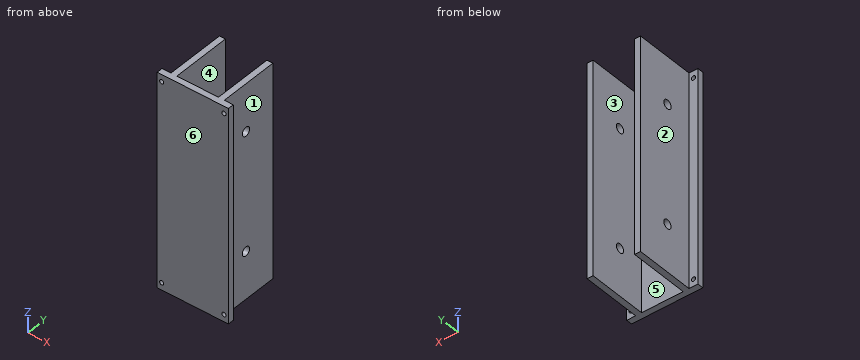
```python
from build123d import *

# Parameters (mm, degrees)
BOSS_EXTRUDE1_DEPTH = 228.6
SKETCH4_R           = 2.2479
CUT_EXTRUDE1_DEPTH  = 250.191994253
SKETCH5_R           = 4.7625
CUT_EXTRUDE2_DEPTH  = 249.158292477


with BuildPart() as part:
    # Sketch1 → Boss-Extrude1 (new body)
    with BuildSketch(Plane.XY):
        Polygon((0, 0), (76.2, 0), (76.2, 6.35), (66.675, 6.35), (66.675, 69.85), (60.325, 69.85), (60.325, 6.35), (15.875, 6.35), (15.875, 69.85), (9.525, 69.85), (9.525, 6.35), (0, 6.35), align=None)
    extrude(amount=BOSS_EXTRUDE1_DEPTH)

    # Sketch4 → Cut-Extrude1 (cut, through all)
    with BuildSketch(Plane(origin=(0, 6.35, 0), x_dir=(1, 0, 0), z_dir=(0, 1, 0))):
        with Locations(Location((4.7625, -7.62, 0), (0, 0, 180))):
            Circle(SKETCH4_R)
        with Locations(Location((4.7625, -220.98, 0), (0, 0, 180))):
            Circle(SKETCH4_R)
        with Locations((71.4375, -220.98)):
            Circle(SKETCH4_R)
        with Locations((71.4375, -7.62)):
            Circle(SKETCH4_R)
    extrude(amount=-CUT_EXTRUDE1_DEPTH, mode=Mode.SUBTRACT)

    # Sketch5 → Cut-Extrude2 (cut, through all)
    with BuildSketch(Plane(origin=(66.675, 0, 0), x_dir=(0, 0, -1), z_dir=(1, 0, 0))):
        with Locations(Location((-177.8, 34.676908919, 0), (0, 0, 90))):
            Circle(SKETCH5_R)
        with Locations(Location((-50.8, 34.676908919, 0), (0, 0, 90))):
            Circle(SKETCH5_R)
    extrude(amount=-CUT_EXTRUDE2_DEPTH, mode=Mode.SUBTRACT)


solid = part.part
```
Geometry: final body of the model. Coordinates: model frame, mm. Face numbers are marked on the shaded views. A direction names the side the tool comes from. Coordinates: 2 decimals unless noted, no trailing zeros. Order: outer loops, then holes, each group sorted by start corner. A loop starts at its lowest first (then second) coordinate and runs counter-clockwise, first axis right, second up. Notation, with made-up numbers: (37.5, -3.5) -> (52.5, -3.5) arc R12 cw to (52.5, 8.5) -> close; hole circle Ø5 at (16.25, -34). An arc over 180 degrees is marked (long way). Write each question's results on one line, items separated by ' | '. Start each with the question number.
1) Cut plane B-B, the plane y = 60. Output: boundary loops of the cut face in (x, z) (3 decimals), and give its area (3 significant figures).
2) First-contact query: pin 1 (5 mm diameter, centred on y = 53, z = 101.5, fed in from -X) (3 decimals); pin 2 (3 mm diameter, centred on x = 20.5, z = 74.5, fed in from +Y); pin 3 (12.5 mm diameter, centred on y = 34.68, z = 50.8, fed in from +X) (3 decimals). Flat tips, straight axial feed; report the tip coordinate or a pass-through.
3) Material intervals for line 1 along X through (y, z) = (3.25, 220.98); line 2 along X through (y, z) = (20, 94.5) (3 decimals); line 3 along Y through (x, z) = (6, 111), sorted ascending.
4) Cut plane D-D, the plane z = 7.62. Output: boundary loops of the cut face in (x, y) (3 decimals), and give its area (3 significant figures).
5) Mould query, pull axis X, two halves, no side actions, for the marked faces 1, 2, 3 and 4. Classes: released by +X, released by -X, zero draft, split by the parting line, or undercut.
6) Cut plane C-C, the plane z = 210. Output: boundary loops of the cut face in (x, y) (3 decimals), and give its area (3 significant figures).
7) Set-up query: the marked faces 5 and 6. Return all of +Z, -Z, +X, -X, +Y, -Y with unobstructed straight access to the full face (end or side cutting, diameter ignored); none if empty.
8) Cut plane A-A, the plane z = 50.8. Output: boundary loops of the cut face in (x, y) (3 decimals), and give its area (3 significant figures).
Checks:
1) outline: (9.525, 0) -> (15.875, 0) -> (15.875, 228.6) -> (9.525, 228.6) -> close; (60.325, 0) -> (66.675, 0) -> (66.675, 228.6) -> (60.325, 228.6) -> close | area: 2,900 mm^2
2) pin 1: x = 9.525 | pin 2: y = 6.35 | pin 3: x = 66.675
3) line 1: 0 to 2.51, 7.01 to 69.19, 73.69 to 76.2 | line 2: 9.525 to 15.875, 60.325 to 66.675 | line 3: 0 to 6.35
4) outline: (0, 0) -> (2.515, 0) -> (2.515, 6.35) -> (0, 6.35) -> close; (7.01, 0) -> (69.19, 0) -> (69.19, 6.35) -> (66.675, 6.35) -> (66.675, 69.85) -> (60.325, 69.85) -> (60.325, 6.35) -> (15.875, 6.35) -> (15.875, 69.85) -> (9.525, 69.85) -> (9.525, 6.35) -> (7.01, 6.35) -> close; (73.685, 0) -> (76.2, 0) -> (76.2, 6.35) -> (73.685, 6.35) -> close | area: 1,230 mm^2
5) face 1: released by +X | face 2: released by -X | face 3: undercut | face 4: undercut
6) outline: (0, 0) -> (76.2, 0) -> (76.2, 6.35) -> (66.675, 6.35) -> (66.675, 69.85) -> (60.325, 69.85) -> (60.325, 6.35) -> (15.875, 6.35) -> (15.875, 69.85) -> (9.525, 69.85) -> (9.525, 6.35) -> (0, 6.35) -> close | area: 1,290 mm^2
7) face 5: +Z, -Z, +Y | face 6: +Z, -Z, +X, -X, -Y
8) outline: (0, 0) -> (76.2, 0) -> (76.2, 6.35) -> (66.675, 6.35) -> (66.675, 29.914) -> (60.325, 29.914) -> (60.325, 6.35) -> (15.875, 6.35) -> (15.875, 29.914) -> (9.525, 29.914) -> (9.525, 6.35) -> (0, 6.35) -> close; (9.525, 39.439) -> (15.875, 39.439) -> (15.875, 69.85) -> (9.525, 69.85) -> close; (60.325, 39.439) -> (66.675, 39.439) -> (66.675, 69.85) -> (60.325, 69.85) -> close | area: 1,170 mm^2
